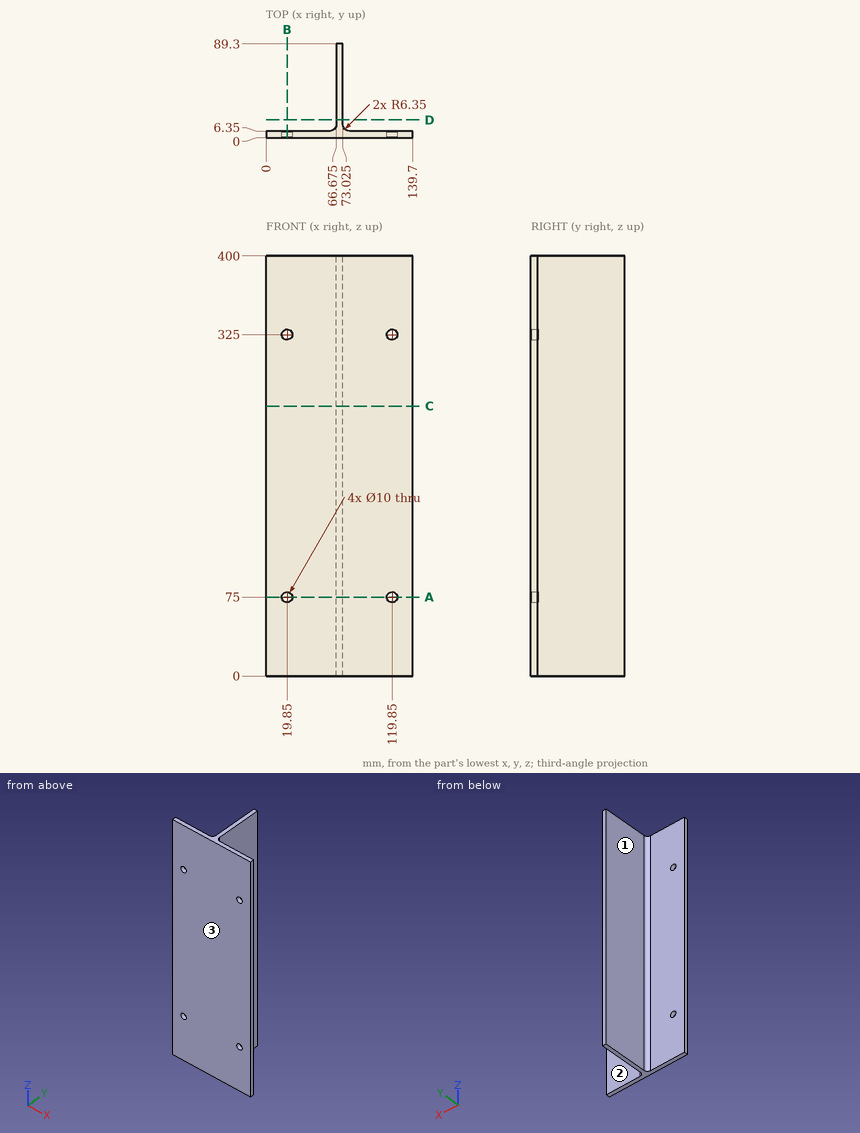
Drawing for the job (mm, zero at the part's lowest x, y, z). A direction names the side the tool comes from. Give positions to 0.01 mm unless a question says otherwise; leave off trailing zeros. Order: outer loops, then holes, each group sorted by start corner. A loop starts at its lowest first (then second) coordinate and runs counter-clockwise, first axis right, second up. Notation, with made-up numbers: M 22,-31.5 L 75,-31.5 A33 cw 75,0.5 Z; hole C 14,80.5 d8. An arc over 180 degrees is marked long. Write item = value, one per line. Start each with the question number.
(1) Which spindle directions (+Z, -Z, +X, -X, +Y, -Y) get a long thin tool onto all of the face, cutting with end or side? Do the marked faces 1, 2 and 3. Say none if no direction does.
(2) Probe L1, parallel to X at y = 3, z = 325; L2, parallel to Z at x = 19.85, y = 5; L3, parallel to Z at x = 119, y = 4. List the from-to ranges inside material, lowest first. Write a range as [from, to].
(3) Slice it at A-A on z = 75. Write the cut outline in (x, y) (3 decimals).
(4) Pin check, flat tips, straight feed: pin 1 Ø6 at (x, z) = (95, 313.5) entering from +Y; pin 2 Ø9 at (x, z) = (19.85, 325) entering from -Y; pin 3 Ø5 at (x, y) = (70, 52) entering from -Z; pin 4 Ø8 at (x, z) = (82.5, 348) entering from +Y. Stop position of each tip, or through.
(5) Slice it at C-C on z = 257. Write the cut outline in (x, y) (3 decimals), plus the area to 3 significant figures.
(6) Slice it at D-D on y = 17. Write the cut outline in (x, z) (3 decimals), plus the area to 3 significant figures.
(7) Slice it at B-B on x = 19.85. Write the cut outline in (y, z).
Responses:
q1.face_1 = +Z, -Z, -X, +Y
q1.face_2 = +Z, -Z, +X, +Y
q1.face_3 = +Z, -Z, +X, -X, -Y
q2.L1 = [0, 14.85], [24.85, 114.85], [124.85, 139.7]
q2.L2 = [0, 70], [80, 320], [330, 400]
q2.L3 = [0, 70.07], [79.93, 320.07], [329.93, 400]
q3.outline = M 0,0 L 14.85,0 L 14.85,6.35 L 0,6.35 Z; M 24.85,0 L 114.85,0 L 114.85,6.35 L 79.375,6.35 A6.35 cw 73.025,12.7 L 73.025,89.3 L 66.675,89.3 L 66.675,12.7 A6.35 cw 60.325,6.35 L 24.85,6.35 Z; M 124.85,0 L 139.7,0 L 139.7,6.35 L 124.85,6.35 Z
q4.pin_1 = 6.35
q4.pin_2 = through
q4.pin_3 = 0
q4.pin_4 = 6.41
q5.outline = M 0,0 L 139.7,0 L 139.7,6.35 L 79.375,6.35 A6.35 cw 73.025,12.7 L 73.025,89.3 L 66.675,89.3 L 66.675,12.7 A6.35 cw 60.325,6.35 L 0,6.35 Z
q5.area = 1,430 mm2
q6.outline = M 66.675,0 L 73.025,0 L 73.025,400 L 66.675,400 Z
q6.area = 2,540 mm2
q7.outline = M 0,0 L 6.35,0 L 6.35,70 L 0,70 Z; M 0,80 L 6.35,80 L 6.35,320 L 0,320 Z; M 0,330 L 6.35,330 L 6.35,400 L 0,400 Z
